Check sheet for the modelled part. Datum: model origin and axes. Units: mm. A direction names the side the tool comes from. Coordinates: 2 decimals unless noted, no trailing zeros. Order: outer loops, then holes, each group sorted by start corner. A loop starts at its lowest first (then second) coordinate and runs counter-clockwise, first axis right, second up.
from build123d import *

# Parameters (mm, degrees)
F1_DEPTH       = 1000
F3_D           = 13.5
F3_DEPTH       = 16
F3_CSINK_D     = 26.88
F3_CSINK_ANGLE = 90
F3_TIP         = 4.0558091784


with BuildPart() as f1:
    # F0 (on Front) → F1 (new body)
    with BuildSketch(Plane.XZ):
        Polygon((-32.8026744276, 16), (-32.8026744276, 0), (117.1973255724, 0), (117.1973255724, 16), (92.1973255724, 16), (92.1973255724, 8), (67.1973255724, 8), (67.1973255724, 16), (42.1973255724, 16), (17.1973255724, 16), (17.1973255724, 8), (-7.8026744276, 8), (-7.8026744276, 16), align=None)
    extrude(amount=F1_DEPTH)

    # F3
    with Locations(Plane.XY.offset(16)):
        with Locations((42.1973255724, -50), (42.1973255724, -350), (42.1973255724, -650), (42.1973255724, -950)):
            CounterSinkHole(F3_D / 2, F3_CSINK_D / 2, depth=F3_DEPTH, counter_sink_angle=F3_CSINK_ANGLE)
            with Locations((0, 0, -(F3_DEPTH + F3_TIP / 2))):  # 118° drill point
                Cone(0, F3_D / 2, F3_TIP, mode=Mode.SUBTRACT)


solid = f1.part
(1) Cross-section at A-A (z = 13.5). Enter the section's corners in (x, y).
Filled in:
outline: (-32.8, -1000) - (-7.8, -1000) - (-7.8, 0) - (-32.8, 0) - close; (17.2, -1000) - (67.2, -1000) - (67.2, 0) - (17.2, 0) - close; (92.2, -1000) - (117.2, -1000) - (117.2, 0) - (92.2, 0) - close; hole circle Ø21.88 at (42.2, -950); hole circle Ø21.88 at (42.2, -650); hole circle Ø21.88 at (42.2, -350); hole circle Ø21.88 at (42.2, -50)
(2) Release check for a two-part mould opening along Y. For faces 1 (the conical face through (47.41, -645.22, 9.63)), 2 (the flat face through (105, -493, 16)), 3 (the flat face through (41, 0, 8)) record: +Y half, -Y half, draft (parallel to the pull), parting line (faces both ways), or undercut.
Filled in:
face 1: undercut
face 2: draft
face 3: +Y half
(3) Thickness scan on probe 1 along X at (y, z) = (-801, 12); probe 2 along X at (y, z) = (-350, 6.75); probe 3 along Y at (x, z) = (40, 3). Record the ranges inside material, lowest first.
Filled in:
probe 1: x = -32.8 to -7.8, 17.2 to 67.2, 92.2 to 117.2
probe 2: x = -32.8 to 35.45, 48.95 to 117.2
probe 3: y = -1000 to -956.38, -943.62 to -656.38, -643.62 to -356.38, -343.62 to -56.38, -43.62 to 0
(4) Tool access check on faces 4 (the flat face through (80, -493, 8)), 5 (the conical face through (43.12, -942.99, 9.63)). Record the directions out of +Z, -Z, +X, -X, +Y, -Y that give a thin tool (end or side, any length) a straight path to the whole face; none if there is none.
Filled in:
face 4: +Z, +Y, -Y
face 5: +Z
(5) Go/stop test with flat-tipped pins: P1, Ø20, axis at x = 80, y = -588, coming from the +Z side; P2, Ø8, axis at x = 42.2, y = -950, coming from the -Z side. Record where each tip stops, or that it passes through.
Filled in:
P1: stops at z = 8
P2: passes through
(6) Cross-section at B-B (y = -576.5). Enter the section's corners in (x, z), and give its area (3 significant figures).
Filled in:
outline: (-32.8, 0) - (117.2, 0) - (117.2, 16) - (92.2, 16) - (92.2, 8) - (67.2, 8) - (67.2, 16) - (17.2, 16) - (17.2, 8) - (-7.8, 8) - (-7.8, 16) - (-32.8, 16) - close
area: 2,000 mm2
